Could you check a few things on this model? Use its own coordinates, in mm. A direction names the side the tool comes from. Give positions to 0.01 mm unless a question says otherwise; leave off trailing zeros. Order: outer loops, then holes, each group sorted by start corner. A loop starts at its lowest first (then second) coordinate and runs counter-clockwise, first axis right, second up. Notation, with made-up numbers: M 2,88 L 27,88 A14 cw 27,102 Z; hole C -39,-29 d7. An arc over 180 degrees is marked long. Answer in a Markdown table with one row per item. Add a question column.
```python
from build123d import *

# Parameters (mm, degrees)
SKETCH1_W              = 166.217523153
SKETCH1_H              = 177.56469515
BOSS_EXTRUDE1_DEPTH    = 2.54
CONVERT_SOLID1_START   = -79.335378531
CONVERT_SOLID1_DEPTH   = 166.217523153
CONVERT_SOLID1_2_DEPTH = 166.217523153
SKETCH9_W              = 138.38791167
SKETCH9_H              = 38.762646995
CUT_EXTRUDE1_DEPTH     = 128.40199345


# Read off the part's stored shape, not the designer's step: Convert-Solid1
with BuildPart() as part:
    # Sketch1 → Boss-Extrude1 (new body)
    with BuildSketch(Plane.XY):
        with Locations((3.773383045, -0.367528123)):
            Rectangle(SKETCH1_W, SKETCH1_H)
    extrude(amount=BOSS_EXTRUDE1_DEPTH)

    # Convert-Solid1 outline → Convert-Solid1 (cut)
    with BuildSketch(Plane.YZ.offset(CONVERT_SOLID1_START)):
        with BuildLine():
            Line((-89.149875698, 0), (-75.067820962, 0))
            ThreePointArc((-75.067820962, 0), (-69.713597874, 1.896751012), (-64.069875698, 2.54))
            Line((-64.069875698, 2.54), (-89.149875698, 2.54))
            Line((-89.149875698, 2.54), (-89.149875698, 0))
        make_face()
        with BuildLine():
            ThreePointArc((61.302819452, 2.54), (67.170718566, 1.897384277), (72.760452717, 0))
            Line((72.760452717, 0), (88.414819452, 0))
            Line((88.414819452, 0), (88.414819452, 2.54))
            Line((88.414819452, 2.54), (61.302819452, 2.54))
        make_face()
    extrude(amount=CONVERT_SOLID1_DEPTH, mode=Mode.SUBTRACT)

    # Convert-Solid1 2 outline → Convert-Solid1 2 (add)
    with BuildSketch(Plane.YZ.offset(CONVERT_SOLID1_START)):
        with BuildLine():
            ThreePointArc((-75.067820962, 0), (-85.339982271, -9.251321871), (-89.149875698, -22.54))
            Line((-89.149875698, -22.54), (-78.387875698, -22.54))
            ThreePointArc((-78.387875698, -22.54), (-74.194230592, -12.415645107), (-64.069875698, -8.222))
            Line((-64.069875698, -8.222), (61.302819452, -8.222))
            ThreePointArc((61.302819452, -8.222), (72.864015325, -13.010804128), (77.652819452, -24.572))
            Line((77.652819452, -24.572), (88.414819452, -24.572))
            ThreePointArc((88.414819452, -24.572), (84.168731823, -10.004550138), (72.760452717, 0))
            Line((72.760452717, 0), (-75.067820962, 0))
        make_face()
    extrude(amount=CONVERT_SOLID1_2_DEPTH)

    # Sketch9 → Cut-Extrude1 (cut, through all)
    with BuildSketch(Plane.XY.offset(2.54)):
        with Locations((5.35195238, 0.49679134)):
            Rectangle(SKETCH9_W, SKETCH9_H)
    extrude(amount=-CUT_EXTRUDE1_DEPTH, mode=Mode.SUBTRACT)


solid = part.part
```
1. Suppose I cut it at B-B on x = 68. List the corners of the cut face in (y, z) for me, plus the area to 3 significant figures.
2. Suppose I cut it at A-A on y = 0. List the corners of the cut face in (x, z) for me, plus the area to 3 significant figures.
3. If I drill on line 1 along X through (y, z) = (-4.5, -3); line 2 along Z through (x, y) = (70, -57); line 3 along Y through (x, z) = (-66, -19.25), over which ranges is the centre line in solid material (lowest first)? Write a range as [from, to].
4. Thinking about a two-plate mould opening in X: for faces 4 (the cylindrical face through (2.61, 72.736, -12.884)), 5 (the flat face through (86.882, -2, -5)), 6 (the flat face through (4, 19.878, -3)), which applies, pulls with the +X half, pulls with the -X half, needs draft (parallel to the pull), parting line crosses it, or undercut?
5. For faces 1 (the cylindrical face through (2.61, -74.305, -12.528)), 2 (the flat face through (74.546, 0, -3)), 3 (the flat face through (3, -84, -22.54)), which set-ups out of +Z, -Z, +X, -X, +Y, -Y let a thin tool reach every point of the face, with its end or its side?
6. Will these pins go through, and if not, where does the flat tip stop? P1, Ø12, axis at y = -45, z = -18.5, coming from the -X side; P2, Ø8, axis at x = 4.5, z = -7, coming from the -Y side; P3, Ø5.5, axis at x = 29, y = -85, coming from the -Z side; P4, Ø8, axis at x = 11.5, z = -9.5, coming from the -Y side.
7. Suppose I cut it at C-C on z = -16.75. List the corners of the cut face in (x, y) for me, plus the area to 3 significant figures.
8. Suppose I cut it at D-D on y = 27.5. List the corners of the cut face in (x, z) for me.
Findings below:
| question | item | result |
|---|---|---|
| 1 | outline | M -89.15,-22.54 L -78.39,-22.54 A14.32 cw -64.07,-8.22 L -18.88,-8.22 L -18.88,2.54 L -64.07,2.54 A25.08 ccw Z; M 19.88,-8.22 L 61.3,-8.22 A16.35 cw 77.65,-24.57 L 88.41,-24.57 A27.11 ccw 61.3,2.54 L 19.88,2.54 Z |
| 1 | area | 1,630 mm2 |
| 2 | outline | M -79.34,-8.22 L -63.84,-8.22 L -63.84,2.54 L -79.34,2.54 Z; M 74.55,-8.22 L 86.88,-8.22 L 86.88,2.54 L 74.55,2.54 Z |
| 2 | area | 300 mm2 |
| 3 | line 1 | [-79.34, -63.84], [74.55, 86.88] |
| 3 | line 2 | [-8.22, 2.54] |
| 3 | line 3 | [-88.93, -78], [76.76, 87.89] |
| 4 | face 4 | needs draft |
| 4 | face 5 | pulls with the +X half |
| 4 | face 6 | undercut |
| 5 | face 1 | -Z, +X, -X |
| 5 | face 2 | +Z, -Z |
| 5 | face 3 | -Z, +X, -X, -Y |
| 6 | P1 | through |
| 6 | P2 | y = -86.34 |
| 6 | P3 | z = -22.54 |
| 6 | P4 | y = -87.46 |
| 7 | outline | M -79.34,-88.47 L 86.88,-88.47 L 86.88,-77.16 L -79.34,-77.16 Z; M -79.34,75.66 L 86.88,75.66 L 86.88,87.26 L -79.34,87.26 Z |
| 7 | area | 3,810 mm2 |
| 8 | outline | M -79.34,-8.22 L 86.88,-8.22 L 86.88,2.54 L -79.34,2.54 Z |
